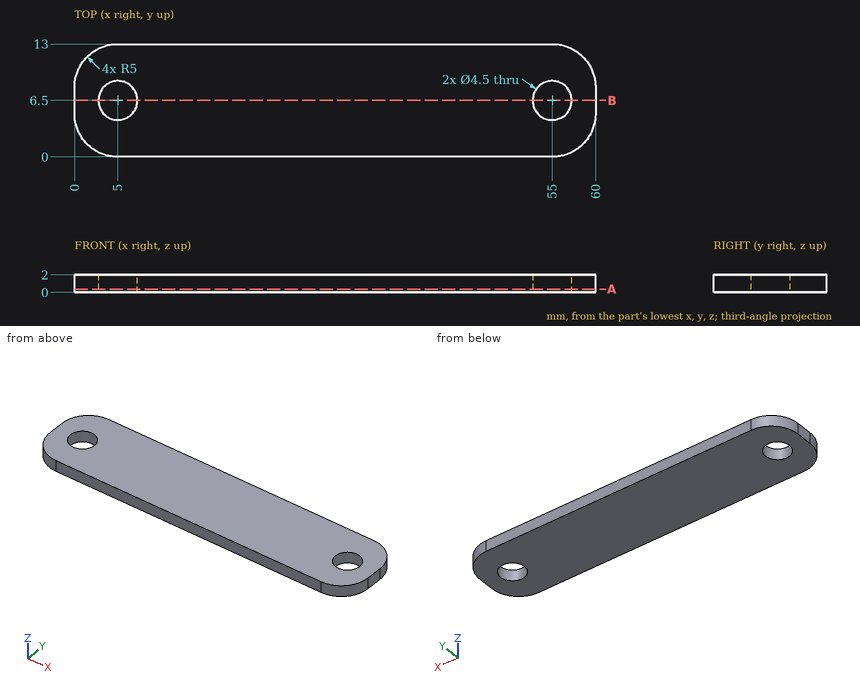
Could you check a few things on this drawing? It's one solid part, dimensions in mm from its lowest x, y, z. Round coordinates to 2 decimals unless told otherwise and drop trailing zeros. Loops run counter-clockwise (first coordinate to the right, second up) from the corner with the lowest first, then second, coordinate; pieces in that order, holes last.
Q1. Please list where these lines run through material, in increasing order: L1, parallel to Y at x = 55, z = 1.2; L2, parallel to X at y = 8.5, z = 1.6; L3, parallel to X at y = 5.5, z = 1.6.
Q2. For P1, Ø1, axis at y = 4.5, z = 1.5, coming from the +X side, with a flat end and sliding along its axis, tell me the tip position at first contact or that it passes through.
Q3. I want a section at B-B (y = 6.5). Write out the boundary of the cut face in (x, z), and give its area (3 significant figures).
Q4. I want a section at A-A (z = 0.35). Write out the boundary of the cut face in (x, y).
Answer below:
1. L1: y = 0 to 4.25, 8.75 to 13
1. L2: x = 0.03 to 3.97, 6.03 to 53.97, 56.03 to 59.97
1. L3: x = 0 to 2.98, 7.02 to 52.98, 57.02 to 60
2. P1: stops at x = 60
3. outline: (0, 0) - (2.75, 0) - (2.75, 2) - (0, 2) - close; (7.25, 0) - (52.75, 0) - (52.75, 2) - (7.25, 2) - close; (57.25, 0) - (60, 0) - (60, 2) - (57.25, 2) - close
3. area: 102 mm2
4. outline: (0, 5) arc R5 ccw to (5, 0) - (55, 0) arc R5 ccw to (60, 5) - (60, 8) arc R5 ccw to (55, 13) - (5, 13) arc R5 ccw to (0, 8) - close; hole circle Ø4.5 at (5, 6.5); hole circle Ø4.5 at (55, 6.5)
